Drawing for the job (mm, zero at the part's lowest x, y, z). A direction names the side the tool comes from. Round coordinates to 2 decimals unless told otherwise and drop trailing zeros. Write each loop counter-clockwise with the first axis right and the second up, starting at its lowest first coordinate (ties: lowest second). Pieces come first, ordered by that corner, then holes.
Item 1: Band-saw the part on D-D, the plane x = 49. Write the cut outline in (y, z).
Item 2: Band-saw the part on A-A, the plane x = 6.5. Write the cut outline in (y, z), then the cut area to 3 significant figures.
Item 3: 3-axis set-ups, long thin cutter, end or side, ignore diameter. For the marked faces 4, 5 and 6: which of +Z, -Z, +X, -X, +Y, -Y reach the whole face in a straight line?
Item 4: Mould opens along Z. For the marked faces 1, 2 and 3 say: +Z half, -Z half, draft (parallel to the pull), parting line (faces both ways), or undercut.
Item 5: Band-saw the part on C-C, the plane z = 4. Write the cut outline in (x, y).
Item 6: Wall check: probe 1 along Y at (x, z) = (21, 37); probe 2 along Z at (x, y) = (10, 43); probe 3 along X at (y, z) = (6, 24). Give the ranges that are in metal, low to high.
Item 7: Band-saw the part on B-B, the plane y = 48. Write the cut outline in (x, z), then the cut area to 4 significant figures.
Item 8: Drop flat-ended pins along their axis: pin 1 Ø16 at (x, y) = (17, 47.5) entering from -Z; pin 2 Ø2 at (y, z) = (8.5, 11.5) entering from -X; pin 3 Ø12 at (x, z) = (24.5, 7.5) entering from -Y; pin 4 Ø10 at (x, y) = (46, 27.5) entering from +Z. Give the stop position or say it passes through.
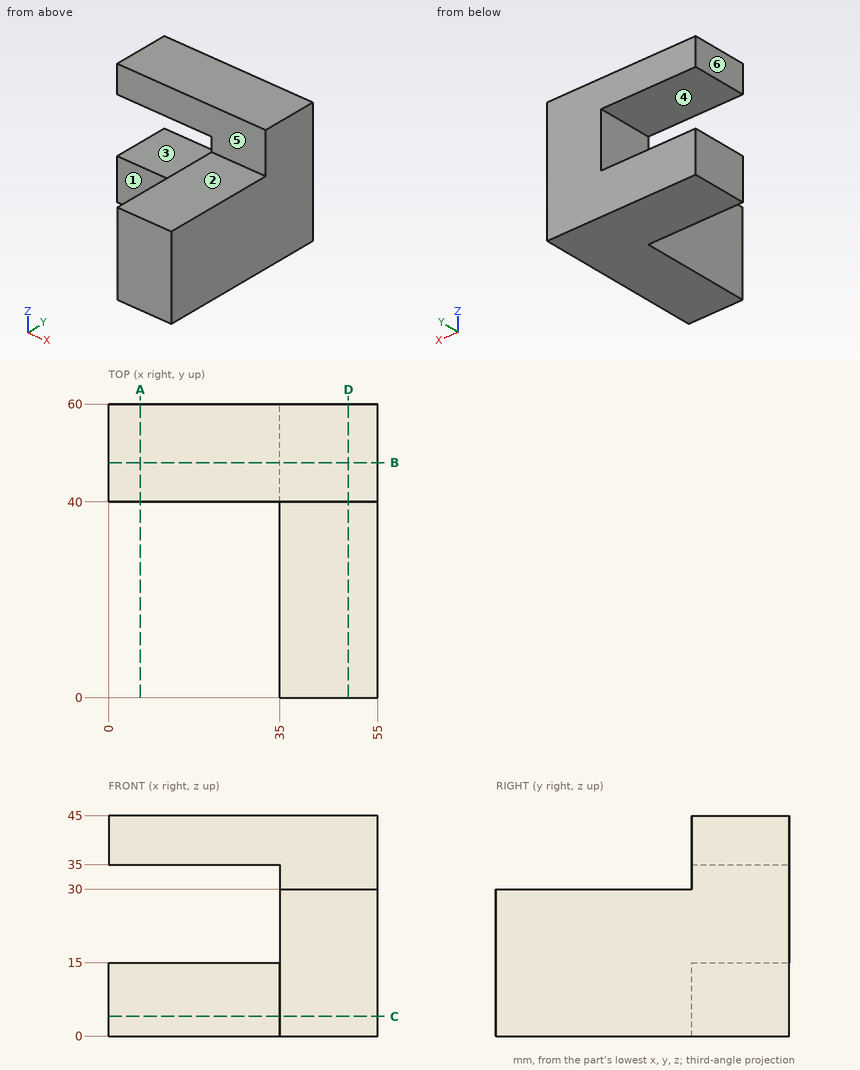
Results:
1. outline: (0, 0) - (60, 0) - (60, 45) - (40, 45) - (40, 30) - (0, 30) - close
2. outline: (40, 0) - (60, 0) - (60, 15) - (40, 15) - close; (40, 35) - (60, 35) - (60, 45) - (40, 45) - close
2. area: 500 mm2
3. face 4: -X, +Y, -Y
3. face 5: +Z, +X, -X, -Y
3. face 6: +Z, -Z, -X, +Y, -Y
4. face 1: draft
4. face 2: +Z half
4. face 3: undercut
5. outline: (0, 40) - (35, 40) - (35, 0) - (55, 0) - (55, 60) - (0, 60) - close
6. probe 1: y = 40 to 60
6. probe 2: z = 0 to 15, 35 to 45
6. probe 3: x = 35 to 55
7. outline: (0, 0) - (55, 0) - (55, 45) - (0, 45) - (0, 35) - (35, 35) - (35, 15) - (0, 15) - close
7. area: 1,775 mm2
8. pin 1: stops at z = 0
8. pin 2: stops at x = 35
8. pin 3: stops at y = 40
8. pin 4: stops at z = 30
